Work out the finished part from the listing and answer in its coordinate system (mm). Face numbers are marked on the shaded views. A direction names the side the tool comes from. Give positions to 0.01 mm unless a question says otherwise; leave off trailing zeros. Order: outer loops, then holes, each group sorted by start corner. A loop starts at its lowest first (then second) coordinate and runs counter-clockwise, first axis right, second up. Notation, with made-up numbers: (68.5, 27.25) - (108.5, 27.25) arc R25 cw to (108.5, 61.25) - close; hole circle Ø1 at (43.25, 2.5). An arc over 180 degrees is marked (long way). Put each result on its own line as item: value.
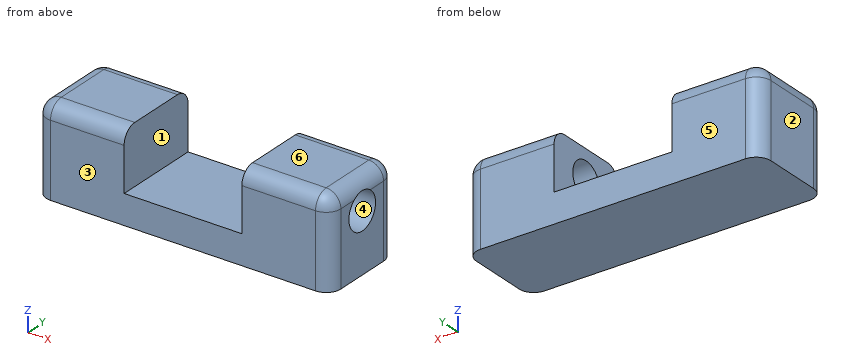
```python
from build123d import *

# Parameters (mm, degrees)
F1_DEPTH     = 60
F2_R         = 12.5
F3_DEPTH     = 70
F4_T1_DEPTH  = 75
F4_T3_DEPTH  = 40
F4_T5_DEPTH  = 75
F4_T7_DEPTH  = 75
F4_S11_W     = 10
F4_S11_H     = 10
F4_T12_DEPTH = 10
F4_S17_W     = 10
F4_S17_H     = 10
F4_T18_DEPTH = 10
F4_S23_W     = 10
F4_S23_H     = 10
F4_T24_DEPTH = 10
F4_S29_W     = 10
F4_S29_H     = 10
F4_T30_DEPTH = 10


# Not quite as in the source:
# - a fillet or chamfer that OpenCascade refuses, or shapes differently, is made with other operations: its cross-section is extruded or revolved along the edge and cut away or added


with BuildPart() as f1:
    # F0 (on Front) → F1 (new body)
    with BuildSketch(Plane.XZ):
        Polygon((0, 60), (0, 0), (200, 0), (200, 60), (140, 60), (140, 20), (60, 20), (60, 60), align=None)
    extrude(amount=F1_DEPTH)

    # F2 (on face) → F3 (cut)
    with BuildSketch(Plane.YZ.offset(200)):
        with Locations((-30, 40)):
            Circle(F2_R)
    extrude(amount=-F3_DEPTH, mode=Mode.SUBTRACT)

    # F4: fillet of radius 10 on 10 edges, made by hand

    # F4_s2 → F4_t1 (cut)
    with BuildSketch(Plane.XY.offset(-25)):
        with BuildLine():
            ThreePointArc((0, -50), (2.9289321881, -57.0710678119), (10, -60))
            Line((10, -60), (0, -60))
            Line((0, -60), (0, -50))
        make_face()
        with BuildLine():
            ThreePointArc((0, -10), (2.9289321881, -2.9289321881), (10, 0))
            Line((10, 0), (0, 0))
            Line((0, 0), (0, -10))
        make_face()
        with BuildLine():
            ThreePointArc((190, -60), (197.0710678119, -57.0710678119), (200, -50))
            Line((200, -50), (200, -60))
            Line((200, -60), (190, -60))
        make_face()
        with BuildLine():
            ThreePointArc((190, 0), (197.0710678119, -2.9289321881), (200, -10))
            Line((200, -10), (200, 0))
            Line((200, 0), (190, 0))
        make_face()
    extrude(amount=F4_T1_DEPTH, mode=Mode.SUBTRACT)

    # F4_s4 → F4_t3 (cut)
    with BuildSketch(Plane.XZ.offset(10)):
        with BuildLine():
            ThreePointArc((0, 50), (2.9289321881, 57.0710678119), (10, 60))
            Line((10, 60), (0, 60))
            Line((0, 60), (0, 50))
        make_face()
        with BuildLine():
            ThreePointArc((200, 50), (197.0710678119, 57.0710678119), (190, 60))
            Line((190, 60), (200, 60))
            Line((200, 60), (200, 50))
        make_face()
    extrude(amount=F4_T3_DEPTH, mode=Mode.SUBTRACT)

    # F4_s6 → F4_t5 (cut)
    with BuildSketch(Plane.YZ.offset(10)):
        with BuildLine():
            ThreePointArc((-10, 60), (-2.9289321881, 57.0710678119), (0, 50))
            Line((0, 50), (0, 60))
            Line((0, 60), (-10, 60))
        make_face()
        with BuildLine():
            ThreePointArc((-50, 60), (-57.0710678119, 57.0710678119), (-60, 50))
            Line((-60, 50), (-60, 60))
            Line((-60, 60), (-50, 60))
        make_face()
    extrude(amount=F4_T5_DEPTH, mode=Mode.SUBTRACT)

    # F4_s8 → F4_t7 (cut)
    with BuildSketch(Plane.YZ.offset(115)):
        with BuildLine():
            ThreePointArc((-60, 50), (-57.0710678119, 57.0710678119), (-50, 60))
            Line((-50, 60), (-60, 60))
            Line((-60, 60), (-60, 50))
        make_face()
        with BuildLine():
            ThreePointArc((0, 50), (-2.9289321881, 57.0710678119), (-10, 60))
            Line((-10, 60), (0, 60))
            Line((0, 60), (0, 50))
        make_face()
    extrude(amount=F4_T7_DEPTH, mode=Mode.SUBTRACT)


with BuildPart() as f4_tool10:
    # F4_s11 → F4_t12 (new body)
    with BuildSketch(Plane.YZ.offset(10)):
        with Locations((-55, 55)):
            Rectangle(F4_S11_W, F4_S11_H)
    extrude(amount=-F4_T12_DEPTH)

    # F4_s13 → F4_t14 (revolve, cut)
    with BuildSketch(Plane(origin=(10, -50, 50), x_dir=(0, 0.7071067812, -0.7071067812), z_dir=(0, 0.7071067812, 0.7071067812))):
        with BuildLine():
            ThreePointArc((0, -10), (10, 0), (0, 10))
            Line((0, 10), (0, -10))
        make_face()
    revolve(axis=Axis((10, -50, 50), (-1, 0, 0)), mode=Mode.SUBTRACT)


with BuildPart() as f1_1:
    add(f1.part)

    # F4_t9: cut F4_tool10
    add(f4_tool10.part, mode=Mode.SUBTRACT)


with BuildPart() as f4_tool16:
    # F4_s17 → F4_t18 (new body)
    with BuildSketch(Plane.YZ.offset(10)):
        with Locations((-5, 55)):
            Rectangle(F4_S17_W, F4_S17_H)
    extrude(amount=-F4_T18_DEPTH)

    # F4_s19 → F4_t20 (revolve, cut)
    with BuildSketch(Plane(origin=(10, -10, 50), x_dir=(0, -0.7071067812, -0.7071067812), z_dir=(0, 0.7071067812, -0.7071067812))):
        with BuildLine():
            ThreePointArc((0, -10), (10, 0), (0, 10))
            Line((0, 10), (0, -10))
        make_face()
    revolve(axis=Axis((10, -10, 50), (-1, 0, 0)), mode=Mode.SUBTRACT)


with BuildPart() as f1_2:
    add(f1_1.part)

    # F4_t15: cut F4_tool16
    add(f4_tool16.part, mode=Mode.SUBTRACT)


with BuildPart() as f4_tool22:
    # F4_s23 → F4_t24 (new body)
    with BuildSketch(Plane.XZ.offset(50)):
        with Locations((195, 55)):
            Rectangle(F4_S23_W, F4_S23_H)
    extrude(amount=F4_T24_DEPTH)

    # F4_s25 → F4_t26 (revolve, cut)
    with BuildSketch(Plane(origin=(190, -50, 50), x_dir=(-0.7071067812, 0, -0.7071067812), z_dir=(-0.7071067812, 0, 0.7071067812))):
        with BuildLine():
            ThreePointArc((0, -10), (10, 0), (0, 10))
            Line((0, 10), (0, -10))
        make_face()
    revolve(axis=Axis((190, -50, 50), (0, -1, 0)), mode=Mode.SUBTRACT)


with BuildPart() as f1_3:
    add(f1_2.part)

    # F4_t21: cut F4_tool22
    add(f4_tool22.part, mode=Mode.SUBTRACT)


with BuildPart() as f4_tool28:
    # F4_s29 → F4_t30 (new body)
    with BuildSketch(Plane.XZ.offset(10)):
        with Locations((195, 55)):
            Rectangle(F4_S29_W, F4_S29_H)
    extrude(amount=-F4_T30_DEPTH)

    # F4_s31 → F4_t32 (revolve, cut)
    with BuildSketch(Plane(origin=(190, -10, 50), x_dir=(-0.7071067812, 0, -0.7071067812), z_dir=(0.7071067812, 0, -0.7071067812))):
        with BuildLine():
            ThreePointArc((0, -10), (10, 0), (0, 10))
            Line((0, 10), (0, -10))
        make_face()
    revolve(axis=Axis((190, -10, 50), (0, 1, 0)), mode=Mode.SUBTRACT)


with BuildPart() as f1_4:
    add(f1_3.part)

    # F4_t27: cut F4_tool28
    add(f4_tool28.part, mode=Mode.SUBTRACT)


solid = f1_4.part
```
(1) A tool of negligible diameter and unlimited length cuts with its end or side. For the marked faces 1 and 2, from which of +Z, -Z, +X, -X, +Y, -Y can it reach the whole face along a straight path? Write none if from no direction.
Geometry check:
face 1: +Z, +Y, -Y
face 2: +Z, -Z, -X, +Y, -Y
(2) Straight lines are drawn through the part: line 1 (Y direction, x = 183, z = 40); line 2 (Z direction, x = 187, y = -30); line 3 (X direction, y = -41, z = 30.5). For each, find the intervals that lie inside material, in ascending order.
Geometry check:
line 1: y = -60 to -42.5, -17.5 to 0
line 2: z = 0 to 27.5, 52.5 to 60
line 3: x = 0 to 60, 140 to 200
(3) Section D-D, the plane y = -30 is taken. Write down the section's boundary in (x, z).
Geometry check:
outline: (0, 0) - (200, 0) - (200, 27.5) - (140, 27.5) - (140, 20) - (60, 20) - (60, 60) - (10, 60) arc R10 ccw to (0, 50) - close; (140, 52.5) - (199.68, 52.5) arc R10 ccw to (190, 60) - (140, 60) - close
(4) Determine the mould class of the marked faces 3, 4, 5 and 6 for opening direction Y: pulls with the +Y half, pulls with the -Y half, needs draft (parallel to the pull), parting line crosses it, or undercut.
Geometry check:
face 3: pulls with the -Y half
face 4: undercut
face 5: pulls with the +Y half
face 6: needs draft
(5) Section B-B, the plane x = 181 is taken. Write down the section's boundary in (y, z).
Geometry check:
outline: (-60, 0) - (0, 0) - (0, 50) arc R10 ccw to (-10, 60) - (-50, 60) arc R10 ccw to (-60, 50) - close; hole circle Ø25 at (-30, 40)
(6) Section A-A, the plane z = 47.5 is taken. Write down the section's boundary in (x, y), then the cut area to 3 significant figures.
Geometry check:
outline: (0, -50) arc R10 ccw to (10, -60) - (60, -60) - (60, 0) - (10, 0) arc R10 ccw to (0, -10) - close; (140, -60) - (190, -60) arc R10 ccw to (200, -50) - (200, -40) - (140, -40) - close; (140, -20) - (200, -20) - (200, -10) arc R10 ccw to (190, 0) - (140, 0) - close
area: 5,910 mm²
(7) Section C-C, the plane z = 23 is taken. Write down the section's boundary in (x, y).
Geometry check:
outline: (0, -50) arc R10 ccw to (10, -60) - (60, -60) - (60, 0) - (10, 0) arc R10 ccw to (0, -10) - close; (140, -60) - (190, -60) arc R10 ccw to (200, -50) - (200, -10) arc R10 ccw to (190, 0) - (140, 0) - close
(8) Given pin 1 (3 mm diameter, centred on y = -17.5, z = 52.5, fed in from -X), flat-ended and moving along its own axis, determine where the tip first touches the part or whether it passes through.
Geometry check:
pin 1: stops at x = 0.05
